Geometry check sheet. Reference: the model listing, model coordinates, mm. Give positions to 0.01 mm unless a question says otherwise; leave off trailing zeros. Write each loop counter-clockwise with the first axis right and the second up, starting at its lowest first coordinate (ties: lowest second). Pieces come first, ordered by that corner, then holes. Notation, with made-up numbers: (-1.75, -37.75) -> (6.25, -37.75) arc R15 ccw to (6.25, -29.75) -> close; hole circle Ø2 at (-31, 89). An arc over 180 degrees is marked (long way). One line per item, written item: value.
from build123d import *

# Parameters (mm, degrees)
SKETCH1_R           = 3.71
SKETCH1_R_2         = 1.925
BOSS_EXTRUDE1_DEPTH = 1.5875
FILLET1_R           = 3
FILLET2_R           = 2
FILLET3_R           = 2


with BuildPart() as part:
    # Sketch1 → Boss-Extrude1 (new body)
    with BuildSketch(Plane(origin=(0, 0, 0), x_dir=(1, 0, 0), z_dir=(0, 1, 0))):
        with BuildLine():
            Line((-25.148871697, 31.27), (-0.825, 31.27))
            Line((-0.825, 31.27), (-0.825, 41.966494574))
            ThreePointArc((-0.825, 41.966494574), (0, 49.02), (0.825, 41.966494574))
            Line((0.825, 41.966494574), (0.825, 31.27))
            Line((0.825, 31.27), (25.148871697, 31.27))
            ThreePointArc((25.148871697, 31.27), (34.235092347, 34.235092347), (31.27, 25.148871697))
            Line((31.27, 25.148871697), (31.27, 0.825))
            Line((31.27, 0.825), (51.966494574, 0.825))
            ThreePointArc((51.966494574, 0.825), (59.02, 0), (51.966494574, -0.825))
            Line((51.966494574, -0.825), (31.27, -0.825))
            Line((31.27, -0.825), (31.27, -25.148871697))
            ThreePointArc((31.27, -25.148871697), (34.235092347, -34.235092347), (25.148871697, -31.27))
            Line((25.148871697, -31.27), (0.825, -31.27))
            Line((0.825, -31.27), (0.825, -41.966494574))
            ThreePointArc((0.825, -41.966494574), (0, -49.02), (-0.825, -41.966494574))
            Line((-0.825, -41.966494574), (-0.825, -31.27))
            Line((-0.825, -31.27), (-25.148871697, -31.27))
            ThreePointArc((-25.148871697, -31.27), (-34.235092347, -34.235092347), (-31.27, -25.148871697))
            Line((-31.27, -25.148871697), (-31.27, -0.825))
            Line((-31.27, -0.825), (-51.966494574, -0.825))
            ThreePointArc((-51.966494574, -0.825), (-59.02, 0), (-51.966494574, 0.825))
            Line((-51.966494574, 0.825), (-31.27, 0.825))
            Line((-31.27, 0.825), (-31.27, 25.148871697))
            ThreePointArc((-31.27, 25.148871697), (-34.235092347, 34.235092347), (-25.148871697, 31.27))
        make_face()
        with Locations(Location((-30.445, 30.445, 0), (0, 0, 270))):
            Circle(SKETCH1_R, mode=Mode.SUBTRACT)
        with Locations(Location((30.445, 30.445, 0), (0, 0, 90))):
            Circle(SKETCH1_R, mode=Mode.SUBTRACT)
        with Locations(Location((30.445, -30.445, 0), (0, 0, 270))):
            Circle(SKETCH1_R, mode=Mode.SUBTRACT)
        with Locations(Location((-30.445, -30.445, 0), (0, 0, 90))):
            Circle(SKETCH1_R, mode=Mode.SUBTRACT)
        with Locations(Location((0, 45.445, 0), (0, 0, 270))):
            Circle(SKETCH1_R_2, mode=Mode.SUBTRACT)
        with Locations(Location((0, -45.445, 0), (0, 0, 90))):
            Circle(SKETCH1_R_2, mode=Mode.SUBTRACT)
        with BuildLine():
            Line((-25.148871697, 29.62), (25.148871697, 29.62))
            ThreePointArc((25.148871697, 29.62), (26.654907653, 26.654907653), (29.62, 25.148871697))
            Line((29.62, 25.148871697), (29.62, -25.148871697))
            ThreePointArc((29.62, -25.148871697), (26.654907653, -26.654907653), (25.148871697, -29.62))
            Line((25.148871697, -29.62), (-25.148871697, -29.62))
            ThreePointArc((-25.148871697, -29.62), (-26.654907653, -26.654907653), (-29.62, -25.148871697))
            Line((-29.62, -25.148871697), (-29.62, 25.148871697))
            ThreePointArc((-29.62, 25.148871697), (-26.654907653, 26.654907653), (-25.148871697, 29.62))
        make_face(mode=Mode.SUBTRACT)
    extrude(amount=BOSS_EXTRUDE1_DEPTH)

    # Fillet1
    fillet1_edges = [part.edges().sort_by_distance(p)[0] for p in [
        (25.148871697, 0.79375, -31.27),
        (31.27, 0.79375, -25.148871697),
        (31.27, 0.79375, 25.148871697),
        (25.148871697, 0.79375, 31.27),
        (-25.148871697, 0.79375, 31.27),
        (-31.27, 0.79375, 25.148871697),
        (-31.27, 0.79375, -25.148871697),
        (-25.148871697, 0.79375, -31.27),
        (-25.148871697, 0.79375, -29.62),
        (-29.62, 0.79375, -25.148871697),
        (-29.62, 0.79375, 25.148871697),
        (-25.148871697, 0.79375, 29.62),
        (25.148871697, 0.79375, 29.62),
        (29.62, 0.79375, 25.148871697),
        (29.62, 0.79375, -25.148871697),
        (25.148871697, 0.79375, -29.62),
    ]]
    fillet(fillet1_edges, radius=FILLET1_R)

    # Fillet2
    fillet2_edges = [part.edges().sort_by_distance(p)[0] for p in [
        (0.825, 0.79375, -31.27),
        (31.27, 0.79375, -0.825),
        (31.27, 0.79375, 0.825),
        (0.825, 0.79375, 31.27),
        (-0.825, 0.79375, 31.27),
        (-31.27, 0.79375, 0.825),
        (-31.27, 0.79375, -0.825),
        (-0.825, 0.79375, -31.27),
    ]]
    fillet(fillet2_edges, radius=FILLET2_R)

    # Fillet3
    fillet3_edges = [part.edges().sort_by_distance(p)[0] for p in [
        (0.825, 0.79375, -41.966494574),
        (51.966494574, 0.79375, -0.825),
        (51.966494574, 0.79375, 0.825),
        (0.825, 0.79375, 41.966494574),
        (-0.825, 0.79375, 41.966494574),
        (-51.966494574, 0.79375, 0.825),
        (-51.966494574, 0.79375, -0.825),
        (-0.825, 0.79375, -41.966494574),
    ]]
    fillet(fillet3_edges, radius=FILLET3_R)


solid = part.part
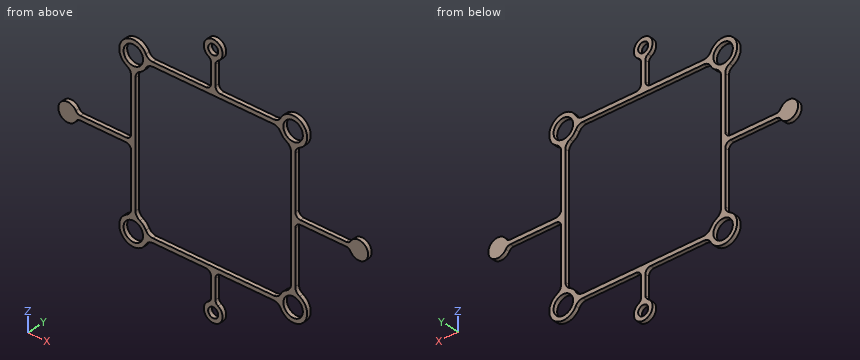
1) Depth check by flat-ended pin: pin 1 Ø0.5 at (x, y) = (4, 0.5) entering from -Z; pin 2 Ø0.8 at (x, y) = (-40, 0.5) entering from +Z (3 decimals); pin 3 Ø0.5 at (x, y) = (11, 0.5) entering from +Z. Enter the tip coordinate at first touch or a pass-through.
Verdict:
pin 1: z = -31.27
pin 2: z = 0.825
pin 3: z = 31.27
2) Sectioned sample at A-A on x = -18.5. Record the cut outline in (y, z).
Verdict:
outline: (0, -31.27) -> (1.59, -31.27) -> (1.59, -29.62) -> (0, -29.62) -> close; (0, 29.62) -> (1.59, 29.62) -> (1.59, 31.27) -> (0, 31.27) -> close
3) Sectioned sample at B-B on y = 1.1. Give the number of separate pieces and of enclosed holes in the cut face, plus the area to 3 significant figures.
Verdict:
separate pieces: 1
enclosed holes: 7
area: 781 mm^2
4) Scan lines: probe 1 along Z at (x, y) = (-30.5, 1.5); probe 2 along Z at (x, y) = (3, 0.4); probe 3 along Z at (x, y) = (30, 1). Record each from-to range of solid material in increasing order.
Verdict:
probe 1: -35.8 to -34.15, -26.74 to 26.74, 34.15 to 35.8
probe 2: -47.39 to -43.5, -31.27 to -29.62, 29.62 to 31.27, 43.5 to 47.39
probe 3: -35.79 to -34.13, -26.76 to 26.76, 34.13 to 35.79
